```python
from build123d import *

# Parameters (mm, degrees)
SKETCH1_R           = 10
BOSS_EXTRUDE1_DEPTH = 25
SKETCH2_R           = 1
BOSS_EXTRUDE2_DEPTH = 10
FILLET1_R           = 2


with BuildPart() as part:
    # Sketch1 → Boss-Extrude1 (new body)
    with BuildSketch(Plane(origin=(0, 0, 0), x_dir=(1, 0, 0), z_dir=(0, 1, 0))):
        Circle(SKETCH1_R)
    extrude(amount=BOSS_EXTRUDE1_DEPTH)

    # Sketch2 → Boss-Extrude2 (add)
    with BuildSketch(Plane(origin=(0, 25, 0), x_dir=(1, 0, 0), z_dir=(0, 1, 0))):
        Circle(SKETCH2_R)
    extrude(amount=BOSS_EXTRUDE2_DEPTH)

    # Fillet1
    fillet1_edges = [part.edges().sort_by_distance(p)[0] for p in [
        (-10, 0, 0),
        (-10, 25, 0),
    ]]
    fillet(fillet1_edges, radius=FILLET1_R)


solid = part.part
```
Can you work these out from the model? Positions are in its coordinate system, mm. A direction names the side the tool comes from. Coordinates: 2 decimals unless noted, no trailing zeros. Write each loop counter-clockwise with the first axis right and the second up, starting at its lowest first coordinate (ties: lowest second). Pieces come first, ordered by that corner, then holes. Notation, with made-up numbers: M 39.5,53 L 53.5,53 A34 cw 53.5,88 Z; hole C 10.25,22 d2. An arc over 180 degrees is marked long. Write item = value, one per line. Start each with the question number.
Q1. If we section it at C-C, the plane y = 18: Write out the boundary of the cut face in (x, z), then the cut area to 3 significant figures.
Q2. If we section it at B-B, the plane x = 0: Write out the boundary of the cut face in (y, z).
Q3. On a 3-axis mill with a long thin cutter (end or side, diameter ignored), from which of +Z, -Z, +X, -X, +Y, -Y can I reach the whole of each face in a straight line? I mean faces 1 (the face through (0, 0, 0)), 2 (the face through (0, 30, 1)). Say none if no direction works.
Q4. I'm going to push flat-ended pins straight in: pin 1 (4 mm diameter, centred on y = 9.5, z = 3.5, fed in from -X); pin 2 (1 mm diameter, centred on y = 13, z = 4.5, fed in from -X); pin 3 (3 mm diameter, centred on y = 16, z = 4, fed in from +X); pin 4 (8 mm diameter, centred on x = -3.5, z = -5, fed in from -Y). Where does each tip first touch, or does it pass through?
Q5. If we section it at D-D, the plane y = 24: Write out the boundary of the cut face in (x, z), then the cut area to 3 significant figures.
Q6. If we section it at A-A, the plane z = 0: Write out the boundary of the cut face in (x, y), then the cut area to 3 significant figures.
Q7. If I drill on L1, parallel to Y at x = 3.75, z = 6.25; L2, parallel to X at y = 2.5, z = -0.25, over which ranges is the centre line in solid material (lowest first)? Write a range as [from, to].
Check sheet entries:
q1.outline = C 0,0 d20
q1.area = 314 mm²
q2.outline = M 0,-8 A2 ccw 2,-10 L 23,-10 A2 ccw 25,-8 L 25,-1 L 35,-1 L 35,1 L 25,1 L 25,8 A2 ccw 23,10 L 2,10 A2 ccw 0,8 Z
q3.face_1 = +Z, -Z, +X, -X, -Y
q3.face_2 = +Y
q4.pin_1 = -9.89
q4.pin_2 = -9.17
q4.pin_3 = 9.68
q4.pin_4 = 0
q5.outline = C 0,0 d19.46
q5.area = 298 mm²
q6.outline = M -10,2 A2 ccw -8,0 L 8,0 A2 ccw 10,2 L 10,23 A2 ccw 8,25 L 1,25 L 1,35 L -1,35 L -1,25 L -8,25 A2 ccw -10,23 Z
q6.area = 517 mm²
q7.L1 = [0, 25]
q7.L2 = [-10, 10]
